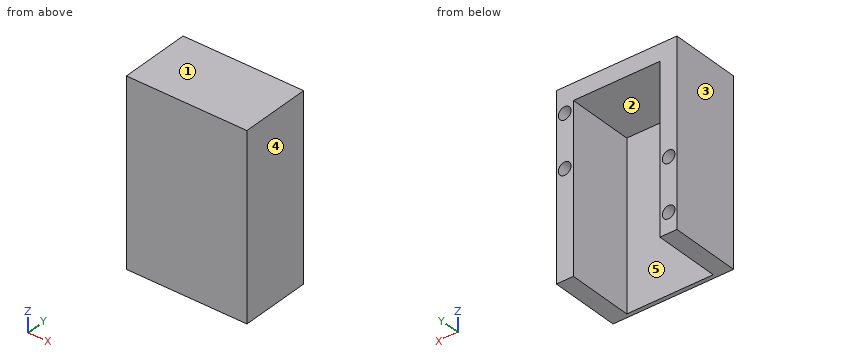
```python
from build123d import *

# Parameters (mm, degrees)
SKETCH1_W                   = 36.83
SKETCH1_H                   = 55.88
BOSS_EXTRUDE1_DEPTH         = 21.59
SKETCH3_W                   = 26.416
SKETCH3_H                   = 20.32
CUT_EXTRUDE1_DEPTH          = 50.8
F_1_0_MM_DOWEL_HOLES1_D     = 3.8608
F_1_0_MM_DOWEL_HOLES1_DEPTH = 5.08
F_1_0_MM_DOWEL_HOLES1_TIP   = 1.159901339


with BuildPart() as part:
    # Sketch1 → Boss-Extrude1 (new body)
    with BuildSketch(Plane(origin=(0, 0, 0), x_dir=(1, 0, 0), z_dir=(0, 1, 0))):
        with Locations((0, 27.94)):
            Rectangle(SKETCH1_W, SKETCH1_H)
    extrude(amount=BOSS_EXTRUDE1_DEPTH)

    # Sketch3 → Cut-Extrude1 (cut)
    with BuildSketch(Plane(origin=(0, 0, -55.88), x_dir=(-1, 0, 0), z_dir=(0, 0, -1))):
        with Locations((0, 11.43)):
            Rectangle(SKETCH3_W, SKETCH3_H)
    extrude(amount=-CUT_EXTRUDE1_DEPTH, mode=Mode.SUBTRACT)

    # Ø1.0 mm Dowel Holes1
    with Locations(Plane(origin=(0, 21.59, 0), x_dir=(1, 0, 0), z_dir=(0, 1, 0))):
        with Locations((15.875, 7.62), (15.875, 23.622), (-15.875, 33.782), (-15.875, 49.784)):
            Hole(F_1_0_MM_DOWEL_HOLES1_D / 2, depth=F_1_0_MM_DOWEL_HOLES1_DEPTH)
            with Locations((0, 0, -(F_1_0_MM_DOWEL_HOLES1_DEPTH + F_1_0_MM_DOWEL_HOLES1_TIP / 2))):  # 118° drill point
                Cone(0, F_1_0_MM_DOWEL_HOLES1_D / 2, F_1_0_MM_DOWEL_HOLES1_TIP, mode=Mode.SUBTRACT)


solid = part.part
```
Input: part model. Units: mm. Frame: model coordinates. Face numbers are marked on the shaded views. A direction names the side the tool comes from. Coordinates: 2 decimals unless noted, no trailing zeros. Order: outer loops, then holes, each group sorted by start corner. A loop starts at its lowest first (then second) coordinate and runs counter-clockwise, first axis right, second up. Notation, with made-up numbers: (-13.5, 26.25) - (-1.5, 26.25) arc R14 cw to (-1.5, 33.25) - close; hole circle Ø3 at (4.25, -11.75). An arc over 180 degrees is marked (long way). Return JSON: item names as keys, results as strings.
Q1. Ray query, probe 1 along X at (y, z) = (12, -46) (3 decimals); probe 2 along X at (y, z) = (18, -8) (3 decimals); probe 3 along Z at (x, y) = (5.5, 1.5). Return the intervals inside material, ascending.
The answers:
{"probe 1": "x = -18.415 to -13.208, 13.208 to 18.415", "probe 2": "x = -18.415 to -13.208, 13.208 to 13.982, 17.768 to 18.415", "probe 3": "z = -5.08 to 0"}
Q2. First-contact query: pin 1 (3 mm diameter, centred on x = -15.875, z = -49.784, fed in from +Y); pin 2 (12 mm diameter, centred on x = -2, y = 13.5, fed in from -Z). Flat tips, straight axial feed; report the tip coordinate or a pass-through.
The answers:
{"pin 1": "stops at y = 16.25", "pin 2": "stops at z = -5.08"}
Q3. Cut plane C-C (y = 18.25). Return loops of the section in (x, z) (3 decimals).
The answers:
{"outline": "(-18.415, -55.88) - (-13.208, -55.88) - (-13.208, -5.08) - (13.208, -5.08) - (13.208, -55.88) - (18.415, -55.88) - (18.415, 0) - (-18.415, 0) - close; hole circle Ø3.861 at (-15.875, -49.784); hole circle Ø3.861 at (-15.875, -33.782); hole circle Ø3.861 at (15.875, -23.622); hole circle Ø3.861 at (15.875, -7.62)"}
Q4. Cut plane A-A (y = 9.25). Return loops of the section in (x, z) (3 decimals), then the cut area to 3 significant figures.
The answers:
{"outline": "(-18.415, -55.88) - (-13.208, -55.88) - (-13.208, -5.08) - (13.208, -5.08) - (13.208, -55.88) - (18.415, -55.88) - (18.415, 0) - (-18.415, 0) - close", "area": "716 mm2"}
Q5. Cut plane B-B (z = -47). Return loops of the section in (x, y) (3 decimals).
The answers:
{"outline": "(-18.415, 0) - (18.415, 0) - (18.415, 21.59) - (13.208, 21.59) - (13.208, 1.27) - (-13.208, 1.27) - (-13.208, 21.59) - (-18.415, 21.59) - close"}
Q6. Access query for the marked faces 1 and 2. Directions: +Z, -Z, +X, -X, +Y, -Y. A direction counts if a zero-diameter tool reaches every point of the face in a straight line with its end or side. Return the directions, or none.
The answers:
{"face 1": "+Z, +X, -X, +Y, -Y", "face 2": "-Z, +Y"}
Q7. Cut plane D-D (x = 9.5). Return loops of the section in (y, z), then the cut area to 3 significant figures.
The answers:
{"outline": "(0, -55.88) - (1.27, -55.88) - (1.27, -5.08) - (21.59, -5.08) - (21.59, 0) - (0, 0) - close", "area": "174 mm2"}
Q8. Draft query along X for the marked faces 3, 4 and 5. Return one class per face: +X half, -X half, draft (parallel to the pull), parting line (faces both ways), or undercut.
The answers:
{"face 3": "-X half", "face 4": "+X half", "face 5": "undercut"}
